Could you check a few things on this model? Use its own coordinates, in mm. A direction names the side the tool comes from. Round coordinates to 2 decimals unless told otherwise and drop trailing zeros. Write each loop counter-clockwise with the first axis right and the second up, starting at its lowest first coordinate (ties: lowest second). Pieces come first, ordered by that corner, then holes. Notation, with made-up numbers: (31, 19.5) -> (49, 19.5) arc R27 ccw to (49, 55.5) -> close; hole circle Ø3 at (41.5, 15). An arc over 180 degrees is marked (long way). Answer as CSV lines item,"result". Start each with the question number.
Q1. Imagine slicing it at B-B on y = 131. Please give me the cut outline in (x, z), and give its area (3 significant figures).
Q2. Imagine slicing it at C-C on z = 31.5. Please give me the cut outline in (x, y).
Q3. Imagine slicing it at A-A on z = 20.5. Please give me the cut outline in (x, y), and give its area (3 significant figures).
Q4. Will these pins go through, and if not, where does the flat tip stop? pin 1 Ø0.9 at (x, z) = (2, -3.5) entering from -Y; pin 2 Ø1.5 at (x, y) = (1.5, 99) entering from -Z; pin 3 Ø1.5 at (x, z) = (2, 26) entering from +Y.
Q5. If we mould it in two halves opening along Y, with no side actions, what happens to faces 1 (the flat face through (1, 50, -6)), 2 (the flat face through (1, 170, 12)), 3 (the flat face through (1, 140, 0))? For each: pulls with the +Y half, pulls with the -Y half, needs draft (parallel to the pull), parting line crosses it, or undercut.
Q6. If I drill on line 1 (Z direction, x = 1.6, y = 100); line 2 (Y direction, x = 0.7, z = 13.5); line 3 (Z direction, x = 2.5, y = 89), over which ranges is the centre line in solid material (lowest first)? Write a range as [from, to].
Q7. For faces 4 (the flat face through (1, 15, 11)), 5 (the flat face through (1, 160, 28)), 6 (the flat face through (1, 85, -3)), 7 (the flat face through (1, 2, 0)), which set-ups out of +Z, -Z, +X, -X, +Y, -Y let a thin tool reach every point of the face, with its end or its side?
Autodesk Fusion 360 part; units mm, degrees
sketch "Sketch1" plane through (0, 0, 0) normal (1, 0, 0) x (0, 1, 0)
  line L0 (0, 0) -> (160, 0)
  line L1 (160, 0) -> (160, 40)
  line L2 (160, 40) -> (0, 40)
  line L3 (0, 40) -> (0, 0)
  line L4 (5, 0) -> (5, -5)
  line L5 (6, -6) -> (14, -6)
  line L6 (15, -5) -> (15, 0)
  line L7 (25, 0) -> (35, 0)
  line L8 (35, 0) -> (35, -5)
  line L9 (34, -6) -> (26, -6)
  line L10 (25, -5) -> (25, 0)
  line L11 (45, 0) -> (55, 0)
  line L12 (55, 0) -> (55, -5)
  line L13 (54, -6) -> (46, -6)
  line L14 (45, -5) -> (45, 0)
  line L15 (65, 0) -> (75, 0)
  line L16 (75, 0) -> (75, -5)
  line L17 (74, -6) -> (66, -6)
  line L18 (65, -5) -> (65, 0)
  line L19 (85, 0) -> (95, 0)
  line L20 (95, 0) -> (95, -5)
  line L21 (94, -6) -> (86, -6)
  line L22 (85, -5) -> (85, 0)
  line L23 (105, 0) -> (115, 0)
  line L24 (115, 0) -> (115, -5)
  line L25 (114, -6) -> (106, -6)
  line L26 (105, -5) -> (105, 0)
  line L27 (125, 0) -> (135, 0)
  line L28 (135, 0) -> (135, -5)
  line L29 (134, -6) -> (126, -6)
  line L30 (125, -5) -> (125, 0)
  line L31 (145, 0) -> (155, 0)
  line L32 (155, 0) -> (155, -5)
  line L33 (154, -6) -> (146, -6)
  line L34 (145, -5) -> (145, 0)
  line L35 (15, -2.5) -> (25, -2.5) construction
  line L36 (35, -2.5) -> (45, -2.5) construction
  line L37 (55, -2.5) -> (65, -2.5) construction
  line L38 (75, -2.5) -> (85, -2.5) construction
  line L39 (95, -2.5) -> (105, -2.5) construction
  line L40 (115, -2.4317) -> (125, -2.4308) construction
  line L41 (135, -2.5) -> (145, -2.5054) construction
  line L42 (10, 0) -> (10, 18)
  line L43 (15, 15) -> (15, 0)
  line L44 (10, 6) -> (15, 6)
  line L45 (10, 18) -> (10, 26)
  line L46 (18, 18) -> (145, 18)
  line L47 (145, 18) -> (145, 29)
  line L48 (145, 29) -> (13, 29)
  line L49 (15, 6) -> (160, 6) construction
  line L50 (145, 18) -> (145, 6) construction
  arc A0 (13, 29) -> (10, 26) centre (13, 26) ccw
  arc A1 (18, 18) -> (15, 15) centre (18, 15) ccw
  line L51 (25, 18) -> (25, 0) construction
  line L52 (160, 14.5) -> (160, 9.5) construction
  line L53 (19.9191, 18) -> (19.9191, 6) construction
  line L54 (160, 7) -> (160, 17) construction
  arc A2 (5, -5) -> (6, -6) centre (6, -5) ccw
  arc A3 (14, -6) -> (15, -5) centre (14, -5) ccw
  arc A4 (25, -5) -> (26, -6) centre (26, -5) ccw
  arc A5 (34, -6) -> (35, -5) centre (34, -5) ccw
  arc A6 (45, -5) -> (46, -6) centre (46, -5) ccw
  arc A7 (54, -6) -> (55, -5) centre (54, -5) ccw
  arc A8 (65, -5) -> (66, -6) centre (66, -5) ccw
  arc A9 (74, -6) -> (75, -5) centre (74, -5) ccw
  arc A10 (85, -5) -> (86, -6) centre (86, -5) ccw
  arc A11 (94, -6) -> (95, -5) centre (94, -5) ccw
  arc A12 (105, -5) -> (106, -6) centre (106, -5) ccw
  arc A13 (114, -6) -> (115, -5) centre (114, -5) ccw
  arc A14 (125, -5) -> (126, -6) centre (126, -5) ccw
  arc A15 (134, -6) -> (135, -5) centre (134, -5) ccw
  arc A16 (145, -5) -> (146, -6) centre (146, -5) ccw
  arc A17 (154, -6) -> (155, -5) centre (154, -5) ccw
  line L55 (160, 17) -> (170, 17)
  line L56 (170, 17) -> (170, 7)
  line L57 (170, 7) -> (160, 7)
  line L58 (160, 7) -> (160, 17)
  line L59 (170, 12) -> (19.9191, 12) construction
  point P0 (5, -6)
  point P1 (15, -6)
  point P2 (15, 18)
  point P3 (10, 29)
  dimension "d1" = 160
  dimension "d2" = 40
  dimension "d3" = 10
  dimension "d4" = 6
  dimension "d5" = 5
  dimension "d6" = 10
  dimension "d7" = 5
  dimension "d9" = 18
  dimension "d10" = 5
  dimension "d15" = 11
  dimension "d16" = 130
  dimension "d17" = 12
  dimension "d18" = 3
  dimension "d19" = 3
  dimension "d29" = 1
  dimension "d30" = 1
  dimension "d31" = 1
  dimension "d32" = 1
  dimension "d33" = 1
  dimension "d34" = 1
  dimension "d35" = 1
  dimension "d36" = 1
  dimension "d37" = 1
  dimension "d38" = 1
  dimension "d39" = 1
  dimension "d40" = 1
  dimension "d41" = 1
  dimension "d42" = 1
  dimension "d43" = 1
  dimension "d44" = 1
  dimension "d45" = 10
  dimension "d46" = 10
extrude "Extrude1" add sketch "Sketch1" along normal blind 3 contours L0 L1 L2 L3 L7 L11 L15 L19 L23 L27 L31 L42 L43 L45 L46 L47 L48 A0 A1 L58 | L0 L4 L5 L6 A2 A3 | L0 L42 L43 L44 | L1 L55 L56 L57 L58 | L0 L7 L8 L9 L10 A4 A5 | L0 L11 L12 L13 L14 A6 A7 | L0 L31 L32 L33 L34 A16 A17 | L0 L15 L16 L17 L18 A8 A9 | L0 L27 L28 L29 L30 A14 A15 | L0 L19 L20 L21 L22 A10 A11 | L0 L23 L24 L25 L26 A12 A13
sketch "Sketch2" plane through (3, 0, 0) normal (1, 0, 0) x (0, 1, 0)
  line L0 (145, 29) -> (145, 18)
  line L1 (145, 18) -> (18, 18)
  arc A0 (18, 18) -> (15, 15) centre (18, 15) ccw
  line L2 (15, 15) -> (15, 6)
  line L3 (15, 6) -> (10, 6)
  line L4 (10, 6) -> (10, 26)
  arc A1 (13, 29) -> (10, 26) centre (13, 26) ccw
  line L5 (13, 29) -> (145, 29)
  line L6 (160, 17) -> (160, 40)
  line L7 (160, 40) -> (0, 40)
  line L8 (0, 40) -> (0, 0)
  line L9 (0, 0) -> (5, 0)
  line L10 (5, 0) -> (5, -5)
  arc A2 (5, -5) -> (6, -6) centre (6, -5) ccw
  line L11 (6, -6) -> (14, -6)
  arc A3 (14, -6) -> (15, -5) centre (14, -5) ccw
  line L12 (15, -5) -> (15, 0)
  line L13 (15, 0) -> (25, 0)
  line L14 (25, 0) -> (25, -5)
  arc A4 (25, -5) -> (26, -6) centre (26, -5) ccw
  line L15 (26, -6) -> (34, -6)
  arc A5 (34, -6) -> (35, -5) centre (34, -5) ccw
  line L16 (35, -5) -> (35, 0)
  line L17 (35, 0) -> (45, 0)
  line L18 (45, 0) -> (45, -5)
  arc A6 (45, -5) -> (46, -6) centre (46, -5) ccw
  line L19 (46, -6) -> (54, -6)
  arc A7 (54, -6) -> (55, -5) centre (54, -5) ccw
  line L20 (55, -5) -> (55, 0)
  line L21 (55, 0) -> (65, 0)
  line L22 (65, 0) -> (65, -5)
  arc A8 (65, -5) -> (66, -6) centre (66, -5) ccw
  line L23 (66, -6) -> (74, -6)
  arc A9 (74, -6) -> (75, -5) centre (74, -5) ccw
  line L24 (75, -5) -> (75, 0)
  line L25 (75, 0) -> (85, 0)
  line L26 (85, 0) -> (85, -5)
  arc A10 (85, -5) -> (86, -6) centre (86, -5) ccw
  line L27 (86, -6) -> (94, -6)
  arc A11 (94, -6) -> (95, -5) centre (94, -5) ccw
  line L28 (95, -5) -> (95, 0)
  line L29 (95, 0) -> (105, 0)
  line L30 (105, 0) -> (105, -5)
  arc A12 (105, -5) -> (106, -6) centre (106, -5) ccw
  line L31 (106, -6) -> (114, -6)
  arc A13 (114, -6) -> (115, -5) centre (114, -5) ccw
  line L32 (115, -5) -> (115, 0)
  line L33 (115, 0) -> (125, 0)
  line L34 (125, 0) -> (125, -5)
  arc A14 (125, -5) -> (126, -6) centre (126, -5) ccw
  line L35 (126, -6) -> (134, -6)
  arc A15 (134, -6) -> (135, -5) centre (134, -5) ccw
  line L36 (135, -5) -> (135, 0)
  line L37 (135, 0) -> (145, 0)
  line L38 (145, 0) -> (145, -5)
  arc A16 (145, -5) -> (146, -6) centre (146, -5) ccw
  line L39 (146, -6) -> (154, -6)
  arc A17 (154, -6) -> (155, -5) centre (154, -5) ccw
  line L40 (155, -5) -> (155, 0)
  line L41 (155, 0) -> (160, 0)
  line L42 (160, 0) -> (160, 7)
  line L43 (160, 7) -> (170, 7)
  line L44 (170, 7) -> (170, 17)
  line L45 (170, 17) -> (160, 17)
Checks:
1,outline,"(0, -6) -> (3, -6) -> (3, 18) -> (0, 18) -> close; (0, 29) -> (3, 29) -> (3, 40) -> (0, 40) -> close"
1,area,"105 mm^2"
2,outline,"(0, 0) -> (3, 0) -> (3, 160) -> (0, 160) -> close"
3,outline,"(0, 0) -> (3, 0) -> (3, 10) -> (0, 10) -> close; (0, 145) -> (3, 145) -> (3, 160) -> (0, 160) -> close"
3,area,"75.0 mm^2"
4,pin 1,"y = 5"
4,pin 2,"z = 0"
4,pin 3,"y = 160"
5,face 1,"needs draft"
5,face 2,"pulls with the +Y half"
5,face 3,"undercut"
6,line 1,"[0, 18], [29, 40]"
6,line 2,"[0, 10], [15, 170]"
6,line 3,"[-6, 18], [29, 40]"
7,face 4,"+X, -X"
7,face 5,"+Z, +X, -X, +Y"
7,face 6,"-Z, +X, -X"
7,face 7,"-Z, +X, -X, -Y"
